Geometry check sheet. Reference: drawing and pictorial views, mm from the part's lowest x, y, z. Coordinates: 2 decimals unless noted, no trailing zeros. Write each loop counter-clockwise with the first axis right and the second up, starting at its lowest first coordinate (ties: lowest second). Pieces come first, ordered by that corner, then holes. Notation, with made-up numbers: (58, 33) -> (93, 33) arc R17 cw to (93, 47) -> close; hole circle Ø2 at (36.25, 26). An arc over 180 degrees is marked (long way). Answer in a Markdown table with one row per item.
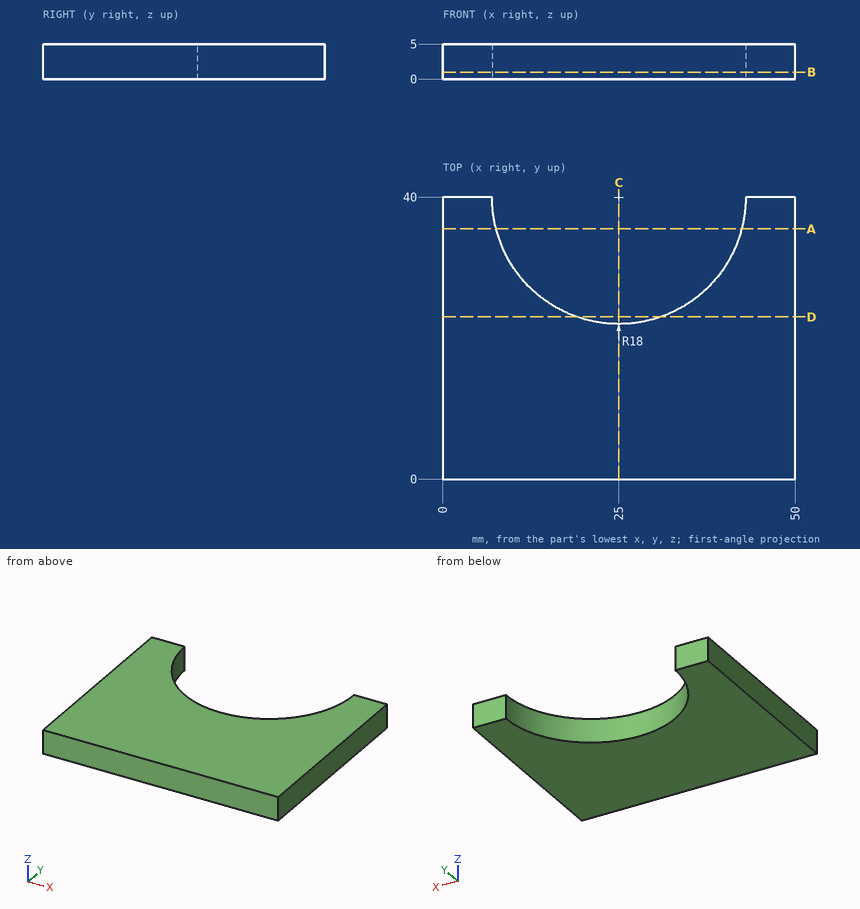
1. Section check D-D, the plane y = 23. Record the boundary of the cut face in (x, z), plus the area to 3 significant figures.
Geometry says:
| item | result |
|---|---|
| outline | (0, 0) -> (19.08, 0) -> (19.08, 5) -> (0, 5) -> close; (30.92, 0) -> (50, 0) -> (50, 5) -> (30.92, 5) -> close |
| area | 191 mm^2 |
2. Section check C-C, the plane x = 25. Record the boundary of the cut face in (y, z), plus the area to 3 significant figures.
Geometry says:
| item | result |
|---|---|
| outline | (0, 0) -> (22, 0) -> (22, 5) -> (0, 5) -> close |
| area | 110 mm^2 |
3. Section check B-B, the plane z = 1. Record the boundary of the cut face in (x, y).
Geometry says:
| item | result |
|---|---|
| outline | (0, 0) -> (50, 0) -> (50, 40) -> (43, 40) arc R18 cw to (7, 40) -> (0, 40) -> close |
4. Thickness scan on line 1 (X direction, y = 38.5, z = 0.35); line 2 (X direction, y = 26, z = 4.75); line 3 (Y direction, x = 25, z = 2.1). Record the ranges inside material, lowest first. Write a range as from..to.
Geometry says:
| item | result |
|---|---|
| line 1 | 0..7.06, 42.94..50 |
| line 2 | 0..13.69, 36.31..50 |
| line 3 | 0..22 |
5. Section check A-A, the plane y = 35.5. Record the boundary of the cut face in (x, z).
Geometry says:
| item | result |
|---|---|
| outline | (0, 0) -> (7.57, 0) -> (7.57, 5) -> (0, 5) -> close; (42.43, 0) -> (50, 0) -> (50, 5) -> (42.43, 5) -> close |
6. Depth check by flat-ended pin: P1, Ø1, axis at y = 31.5, z = 0.5, coming from the -X side. Enter the tip coordinate at first touch or a pass-through.
Geometry says:
| item | result |
|---|---|
| P1 | x = 0 |
